Geometry: final body of the model. Coordinates: model frame, mm. Round coordinates to 2 decimals unless told otherwise and drop trailing zeros. Order: outer loops, then holes, each group sorted by start corner. A loop starts at its lowest first (then second) coordinate and runs counter-clockwise, first axis right, second up. Notation, with made-up numbers: (12.5, 26.5) -> (24.5, 26.5) arc R14 ccw to (24.5, 34.5) -> close; hole circle Ø6 at (88.25, -11). An arc over 180 degrees is marked (long way). Put each result on its own line as item: value.
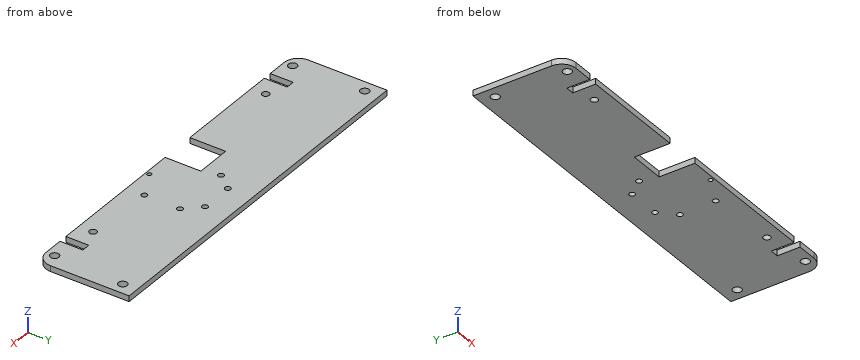
```python
from build123d import *

# Parameters (mm, degrees)
SKETCH1_W           = 260
SKETCH1_H           = 65
BOSS_EXTRUDE2_DEPTH = 4
SKETCH3_R           = 3
CUT_EXTRUDE2_DEPTH  = 135.060620616
FILLET1_R           = 10
SKETCH4_W           = 25
SKETCH4_H           = 25
CUT_EXTRUDE3_DEPTH  = 10
SKETCH5_W           = 6
SKETCH5_H           = 16
CUT_EXTRUDE4_DEPTH  = 135.060620616
SKETCH6_R           = 2.5
CUT_EXTRUDE5_DEPTH  = 135.060620616
SKETCH7_R           = 2
SKETCH7_R_2         = 1.5
CUT_EXTRUDE6_DEPTH  = 10


with BuildPart() as part:
    # Sketch1 → Boss-Extrude2 (new body)
    with BuildSketch(Plane.XY):
        Rectangle(SKETCH1_W, SKETCH1_H)
    extrude(amount=BOSS_EXTRUDE2_DEPTH)

    # Sketch3 → Cut-Extrude2 (cut, through all)
    with BuildSketch(Plane(origin=(0, 0, 0), x_dir=(-1, 0, 0), z_dir=(0, 0, -1))):
        with Locations((120, -26.5)):
            Circle(SKETCH3_R)
        with Locations((-120, -26.5)):
            Circle(SKETCH3_R)
        with Locations((-122, 22.5)):
            Circle(SKETCH3_R)
        with Locations((122, 22.5)):
            Circle(SKETCH3_R)
    extrude(amount=-CUT_EXTRUDE2_DEPTH, mode=Mode.SUBTRACT)

    # Fillet1
    fillet1_edges = [part.edges().sort_by_distance(p)[0] for p in [
        (130, -32.5, 2),
        (-130, -32.5, 2),
    ]]
    fillet(fillet1_edges, radius=FILLET1_R)

    # Sketch4 → Cut-Extrude3 (cut)
    with BuildSketch(Plane(origin=(0, 0, 0), x_dir=(-1, 0, 0), z_dir=(0, 0, -1))):
        with Locations((12.5, -20)):
            Rectangle(SKETCH4_W, SKETCH4_H)
    extrude(amount=-CUT_EXTRUDE3_DEPTH, mode=Mode.SUBTRACT)

    # Sketch5 → Cut-Extrude4 (cut, through all)
    with BuildSketch(Plane(origin=(0, 0, 0), x_dir=(-1, 0, 0), z_dir=(0, 0, -1))):
        with Locations((-103, -24.5)):
            Rectangle(SKETCH5_W, SKETCH5_H)
        with Locations((103, -24.5)):
            Rectangle(SKETCH5_W, SKETCH5_H)
    extrude(amount=-CUT_EXTRUDE4_DEPTH, mode=Mode.SUBTRACT)

    # Sketch6 → Cut-Extrude5 (cut, through all)
    with BuildSketch(Plane(origin=(0, 0, 0), x_dir=(-1, 0, 0), z_dir=(0, 0, -1))):
        with Locations((87.05, -22.5)):
            Circle(SKETCH6_R)
        with Locations((-87.05, -22.5)):
            Circle(SKETCH6_R)
    extrude(amount=-CUT_EXTRUDE5_DEPTH, mode=Mode.SUBTRACT)

    # Sketch7 → Cut-Extrude6 (cut)
    with BuildSketch(Plane(origin=(0, 0, 0), x_dir=(-1, 0, 0), z_dir=(0, 0, -1))):
        with Locations((-39, -20)):
            Circle(SKETCH7_R)
        with Locations((-39, 5)):
            Circle(SKETCH7_R)
        with Locations((-29, 15.5)):
            Circle(SKETCH7_R)
        with Locations((-6, 15.5)):
            Circle(SKETCH7_R)
        with Locations((3, 4.5)):
            Circle(SKETCH7_R)
        with Locations((-19.5, -30)):
            Circle(SKETCH7_R_2)
    extrude(amount=-CUT_EXTRUDE6_DEPTH, mode=Mode.SUBTRACT)


solid = part.part
```
1. Material intervals for probe 1 along X at (y, z) = (23, 3.65); probe 2 along Y at (x, z) = (120, 3); probe 3 along Y at (x, z) = (87.05, 3.15), sorted ascending.
Ans:
probe 1: -130 to -124.96, -119.04 to 119.04, 124.96 to 130
probe 2: -32.5 to -29.5, -23.5 to 20.26, 24.74 to 32.5
probe 3: -32.5 to -25, -20 to 32.5
2. Cut plane A-A on z = 1.1. State how many separate pieces and enclosed holes the cut face has, and give its area (3 significant figures).
Ans:
separate pieces: 1
enclosed holes: 12
area: 15,800 mm²
3. Cut plane B-B on x = 87.05. Return loops of the section in (y, z), and give its area (3 significant figures).
Ans:
outline: (-32.5, 0) -> (-25, 0) -> (-25, 4) -> (-32.5, 4) -> close; (-20, 0) -> (32.5, 0) -> (32.5, 4) -> (-20, 4) -> close
area: 240 mm²
4. Contact query for flat-ended pins moving along their axis: P1, Ø3.5, axis at x = -120, y = -26.5, coming from the +Z side; P2, Ø2, axis at y = -26.5, z = 2.5, coming from the +X side; P3, Ø2, axis at y = -24, z = 2.5, coming from the +X side; P4, Ø2, axis at y = -26, z = 1.5, coming from the -X side. Output: stop coordinate, or through.
Ans:
P1: through
P2: x = 129.54
P3: x = 129.99
P4: x = -129.68
5. Cut plane C-C on x = -19. Return loops of the section in (y, z).
Ans:
outline: (-7.5, 0) -> (32.5, 0) -> (32.5, 4) -> (-7.5, 4) -> close
